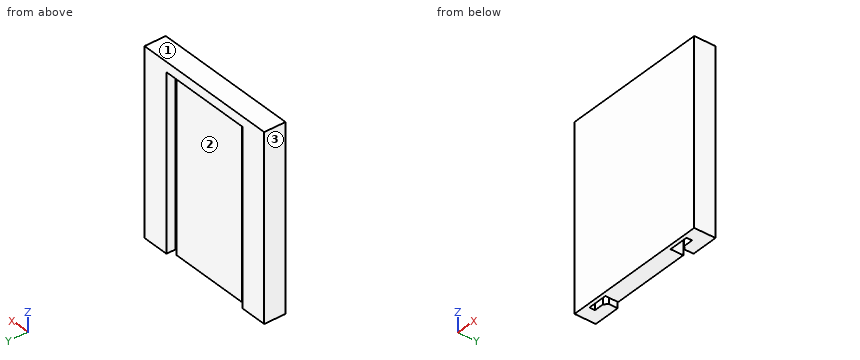
Autodesk Inventor part; units mm, degrees
ref_plane "YZ Plane" through (0, 0, 0) normal (1, 0, 0) x (0, 1, 0)
ref_plane "XZ Plane" through (0, 0, 0) normal (0, 1, 0) x (-1, 0, 0)
ref_plane "XY Plane" through (0, 0, 0) normal (0, 0, 1) x (1, 0, 0)
sketch "Sketch1" plane through (0, 0, 0) normal (0, 0, 1) x (1, 0, 0)
  line L0 (-22.5, 0) -> (22.5, 0)
  line L1 (22.5, 0) -> (22.5, 6.5)
  line L2 (22.5, 6.5) -> (14.25, 6.5)
  line L3 (14.25, 6.5) -> (14.25, 3.8111)
  line L4 (15.25, 2.8111) -> (18.25, 2.8111)
  line L5 (18.25, 2.8111) -> (18.25, 1.1111)
  line L6 (18.25, 1.1111) -> (12.25, 1.1111)
  line L7 (12.25, 1.1111) -> (12.25, 5)
  line L8 (12.25, 5) -> (-12.25, 5)
  line L9 (-12.25, 5) -> (-12.25, 1.1111)
  line L10 (-12.25, 1.1111) -> (-18.25, 1.1111)
  line L11 (-18.25, 1.1111) -> (-18.25, 2.8111)
  line L12 (-18.25, 2.8111) -> (-15.25, 2.8111)
  line L13 (-14.25, 3.8111) -> (-14.25, 6.5)
  line L14 (-14.25, 6.5) -> (-22.5, 6.5)
  line L15 (-22.5, 6.5) -> (-22.5, 0)
  line L16 (15.25, 2.8111) -> (14.25, 3.8111)
  line L17 (-14.25, 3.8111) -> (-15.25, 2.8111)
  point P0 (0, 0)
  point P1 (14.25, 2.8111)
  point P2 (-14.25, 2.8111)
  dimension "d0" = 45
  dimension "d1" = 6.5
  dimension "d2" = 22.5
  dimension "d3" = 36.5
  dimension "d4" = 4.25
  dimension "d5" = 6
  dimension "d6" = 4
  dimension "d7" = 4
  dimension "d8" = 6
  dimension "d9" = 5
  dimension "d14" = 1.1111
  dimension "d15" = 1.7
  dimension "d16" = 1
  dimension "d17" = 1
  dimension "d18" = 1
  dimension "d19" = 1
extrude "Extrusion1" add sketch "Sketch1" along normal blind 53
sketch "Sketch2" plane through (0, 0, 53) normal (0, 0, 1) x (1, 0, 0)
  line L0 (-22.5, 0) -> (22.5, 0)
  line L1 (-22.5, 6.5) -> (-22.5, 0)
  line L2 (22.5, 0) -> (22.5, 6.5)
  line L3 (-22.5, 6.5) -> (22.5, 6.5)
  point P0 (0, 0)
extrude "Extrusion2" add sketch "Sketch2" along normal blind 3
properties part number "placa_metal"
The model under review builds one solid part; all positions refer to its coordinate system, in mm. Face numbers are marked on the shaded views. Round coordinates to 2 decimals unless told otherwise and drop trailing zeros. Loops run counter-clockwise (first coordinate to the right, second up) from the corner with the lowest first, then second, coordinate; pieces in that order, holes last. Notation, with made-up numbers: (59, 84.5) - (75, 84.5) arc R18 ccw to (75, 90.5) - close; hole circle Ø7 at (-19, -6). An arc over 180 degrees is marked (long way). Write each question's results on one line, items separated by ' | '. Start each with the question number.
Q1. Wall thickness on line 1 along X through (y, z) = (1.5, 21); line 2 along X through (y, z) = (4, 32.5); line 3 along Z through (x, y) = (-12, 5.5): over which ranges is each line inside the solid? List them lowest first. Write a range as [from, to].
Q2. Draft analysis for pull direction X (two halves, no side actions). For the marked faces 1, 2 and 3, state which applies: pulls with the +X half, pulls with the -X half, needs draft (parallel to the pull), parting line crosses it, or undercut.
Q3. Insertion check: P1, Ø6, axis at x = 6, z = 24, coming from the +Y side. The pin has a flat end and moves straight along its axis. Give the tip position at first contact, or say it passes through.
Q4. Take a section at B-B on x = -3. Give the boundary of the cut face in (y, z).
Q5. Take a section at A-A on z = 41. Give the boundary of the cut face in (x, y), plus the area to 3 significant figures.
Data:
1) line 1: x = [-22.5, -18.25], [-12.25, 12.25], [18.25, 22.5] | line 2: x = [-22.5, -14.25], [-12.25, 12.25], [14.25, 22.5] | line 3: z = [53, 56]
2) face 1: needs draft | face 2: undercut | face 3: pulls with the -X half
3) P1: stops at y = 5
4) outline: (0, 0) - (5, 0) - (5, 53) - (6.5, 53) - (6.5, 56) - (0, 56) - close
5) outline: (-22.5, 0) - (22.5, 0) - (22.5, 6.5) - (14.25, 6.5) - (14.25, 3.81) - (15.25, 2.81) - (18.25, 2.81) - (18.25, 1.11) - (12.25, 1.11) - (12.25, 5) - (-12.25, 5) - (-12.25, 1.11) - (-18.25, 1.11) - (-18.25, 2.81) - (-15.25, 2.81) - (-14.25, 3.81) - (-14.25, 6.5) - (-22.5, 6.5) - close | area: 220 mm²
